For this review, take the finished solid that the model builds, in its own axes (mm). Face numbers are marked on the shaded views. A direction names the side the tool comes from. Give positions to 0.01 mm unless a question says otherwise; leave off trailing zeros. Write each loop counter-clockwise with the first axis right and the second up, starting at its lowest first coordinate (ties: lowest second). Pieces come first, ordered by that corner, then holes. Notation, with made-up numbers: (-9.75, 66) -> (45.25, 66) arc R13 ccw to (45.25, 89) -> close; hole circle Ø5 at (55.5, 39). An arc over 180 degrees is marked (long way). Write item = value, one per line.
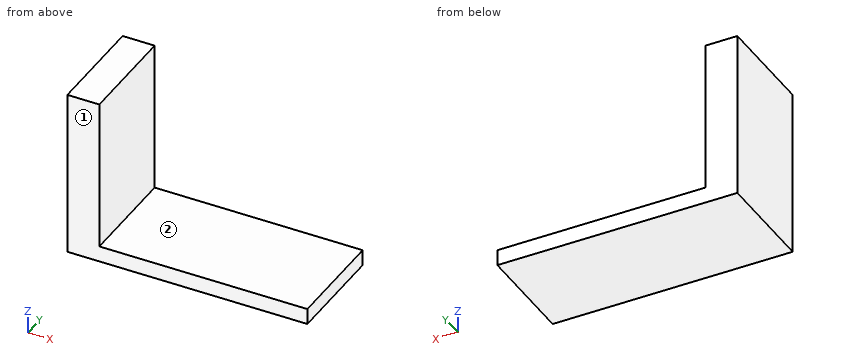
```python
from build123d import *

# Parameters (mm, degrees)
F1_DEPTH  = 25.4
F2_DEPTH  = 57.15
F2_FACE_W = 25.4
F2_FACE_H = 82.55
F3_DEPTH  = 76.2


with BuildPart() as f1:
    # F0 (on Front) → F1 (new body)
    with BuildSketch(Plane.XZ):
        Polygon((0, 57.15), (0, 0), (190.5, 0), (190.5, 12.7), (25.4, 12.7), (25.4, 57.15), align=None)
    extrude(amount=F1_DEPTH)

    # F1_face (on face) → F2 (join)
    with BuildSketch(Plane(origin=(68.984091, -25.4, 15.442045), x_dir=(1, 0, 0), z_dir=(0, -1, 0))):
        Polygon((-43.584091, -2.742045), (-43.584091, 41.707955), (-68.984091, 41.707955), (-68.984091, -15.442045), (121.515909, -15.442045), (121.515909, -2.742045), align=None)
    extrude(amount=F2_DEPTH)

    # F2_face (on face) → F3 (join)
    with BuildSketch(Plane(origin=(12.7, -41.275, 57.15), x_dir=(1, 0, 0), z_dir=(0, 0, 1))):
        Rectangle(F2_FACE_W, F2_FACE_H)
    extrude(amount=F3_DEPTH)


solid = f1.part
```
(1) To check wall thickness, follow probe 1 along X at (y, z) = (-52, 16); probe 2 along Z at (x, y) = (44, -14). State the ranges of each line that lie inside material, in increasing order.
Answers below:
probe_1 = 0 to 25.4
probe_2 = 0 to 12.7
(2) Take a section at C-C (z = 93). Write out the cut boundary in (x, y).
Answers below:
outline = (0, -82.55) -> (25.4, -82.55) -> (25.4, 0) -> (0, 0) -> close
(3) For pin 1 (8 mm diameter, centred on x = 120.5, y = -58, fed in from +Z), flat-tipped, find the tip position at first contact; note if it passes through.
Answers below:
pin_1 = 12.7
(4) Take a section at A-A (y = -17). Write out the cut boundary in (x, z), plus the area to 3 significant figures.
Answers below:
outline = (0, 0) -> (190.5, 0) -> (190.5, 12.7) -> (25.4, 12.7) -> (25.4, 133.35) -> (0, 133.35) -> close
area = 5,480 mm^2
(5) Tool access review of the marked faces 1 and 2: name each direction out of +Z, -Z, +X, -X, +Y, -Y from which nothing blocks a thin tool from reaching the whole face with its end or side.
Answers below:
face_1 = +Z, -Z, +X, -X, -Y
face_2 = +Z, +X, +Y, -Y
(6) Take a section at B-B (x = 79.5). Write out the cut boundary in (y, z).
Answers below:
outline = (-82.55, 0) -> (0, 0) -> (0, 12.7) -> (-82.55, 12.7) -> close
